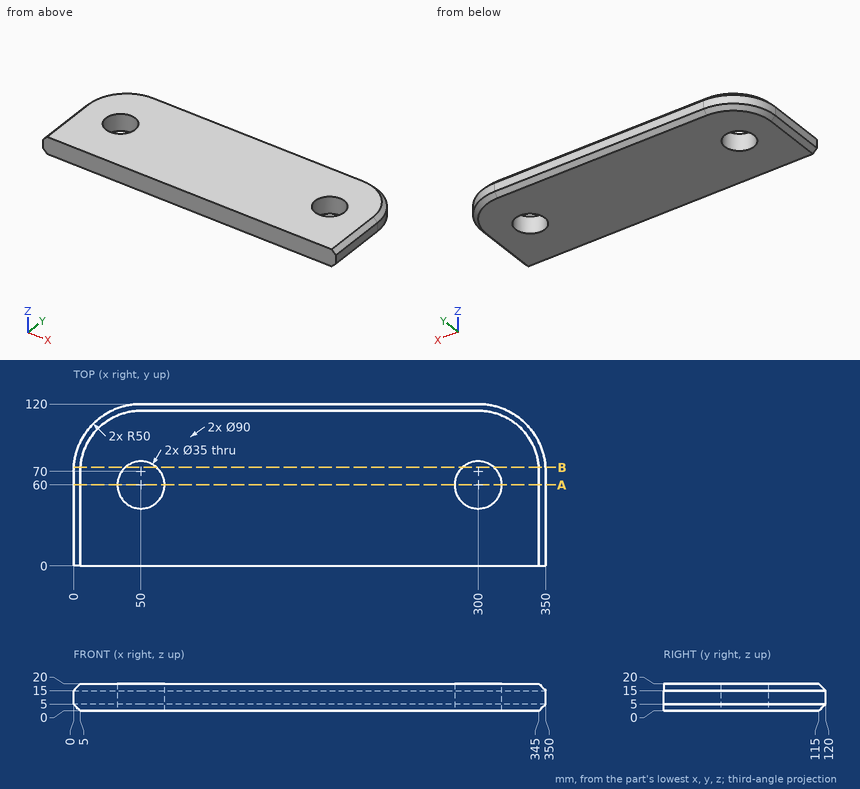
For this review, use the dimensioned drawing (mm, ordinates from the lowest corner) and the shaded views. Round coordinates to 2 decimals unless told otherwise and drop trailing zeros. Write each loop counter-clockwise with the first axis right and the second up, starting at its lowest first coordinate (ties: lowest second). Pieces come first, ordered by that corner, then holes. Notation, with made-up numbers: M -37,64 L -32,64 A22 cw -32,81 Z; hole C -9.75,80.5 d9. An arc over 180 degrees is marked long. Use CSV: the item, a comma, the result in double quotes. Start each with the question number.
(1) For line 1 along Y through (x, z) = (50, 9.5); line 2 along X through (y, z) = (45.5, 12); line 3 along X through (y, z) = (62, 13.25), list the stretches that pass through material, from the lowest coordinate up.
(2) We need section A-A, the plane y = 60. State the section outline as (x, z) points, then the cut area to 3 significant figures.
(3) We need section B-B, the plane y = 73. State how many separate pieces and enclosed holes the cut face has, then the cut area to 3 significant figures.
(4) Clearance check with a flat-ended pin moving along its axis: P1, Ø1.5, axis at y = 20, z = 17.5, coming from the -X side. State where the tip first meets the part, or that it passes through.
Findings:
1,line 1,"0 to 42.5, 77.5 to 120"
1,line 2,"0 to 40.2, 59.8 to 290.2, 309.8 to 350"
1,line 3,"0 to 32.61, 67.39 to 282.61, 317.39 to 350"
2,outline,"M 0,5 L 5,0 L 32.5,0 L 32.5,20 L 5,20 L 0,15 Z; M 67.5,0 L 282.5,0 L 282.5,20 L 67.5,20 Z; M 317.5,0 L 345,0 L 350,5 L 350,15 L 345,20 L 317.5,20 Z"
2,area,"5,550 mm^2"
3,separate pieces,"3"
3,enclosed holes,"0"
3,area,"6,010 mm^2"
4,P1,"x = 1.75"
